Check sheet for the drawn part. Datum: minimum x, y, z corner. Units: mm. A direction names the side the tool comes from. Give positions to 0.01 mm unless a question says otherwise; leave off trailing zeros. Loops run counter-clockwise (first coordinate to the right, second up) from the corner with the lowest first, then second, coordinate; pieces in that order, holes last. Notation, with made-up numbers: (86, 39.5) - (121, 39.5) arc R19 cw to (121, 66.5) - close; hole circle Ø4 at (-26.5, -9). An arc over 180 degrees is marked (long way). Use a Markdown table: item, result. Add a question column.
1. Cross-section at C-C on y = 3.5. Enter the section's corners in (x, z).
2. Depth check by flat-ended pin: P1, Ø2, axis at y = 17, z = 12.5, coming from the -X side; P2, Ø1, axis at y = 8.5, z = 3, coming from the -X side; P3, Ø2, axis at y = 11.5, z = 20, coming from the +X side. Enter the tip coordinate at first touch or a pass-through.
3. Material ranges on L1, parallel to Z at x = 13.97, y = 9.75; L2, parallel to Y at x = 1.5, z = 10.75; L3, parallel to Z at x = 7.5, y = 19.5, recorded low to high.
4. Cross-section at B-B on x = 13.97. Enter the section's corners in (y, z).
5. Cross-section at A-A on z = 13.97. Enter the section's corners in (x, y), and give its area (3 significant figures).
6. Set-up check for the marked faces 4 and 5: record each of +Z, -Z, +X, -X, +Y, -Y from which the full face is reachable in a straight line by a thin tool's end or side.
7. Draft check along X on the marked faces 1, 2 and 3. Enter one of: pulls with the +X half, pulls with the -X half, needs draft (parallel to the pull), parting line crosses it, or undercut.
8. Cross-section at D-D on x = 25. Enter the section's corners in (y, z).
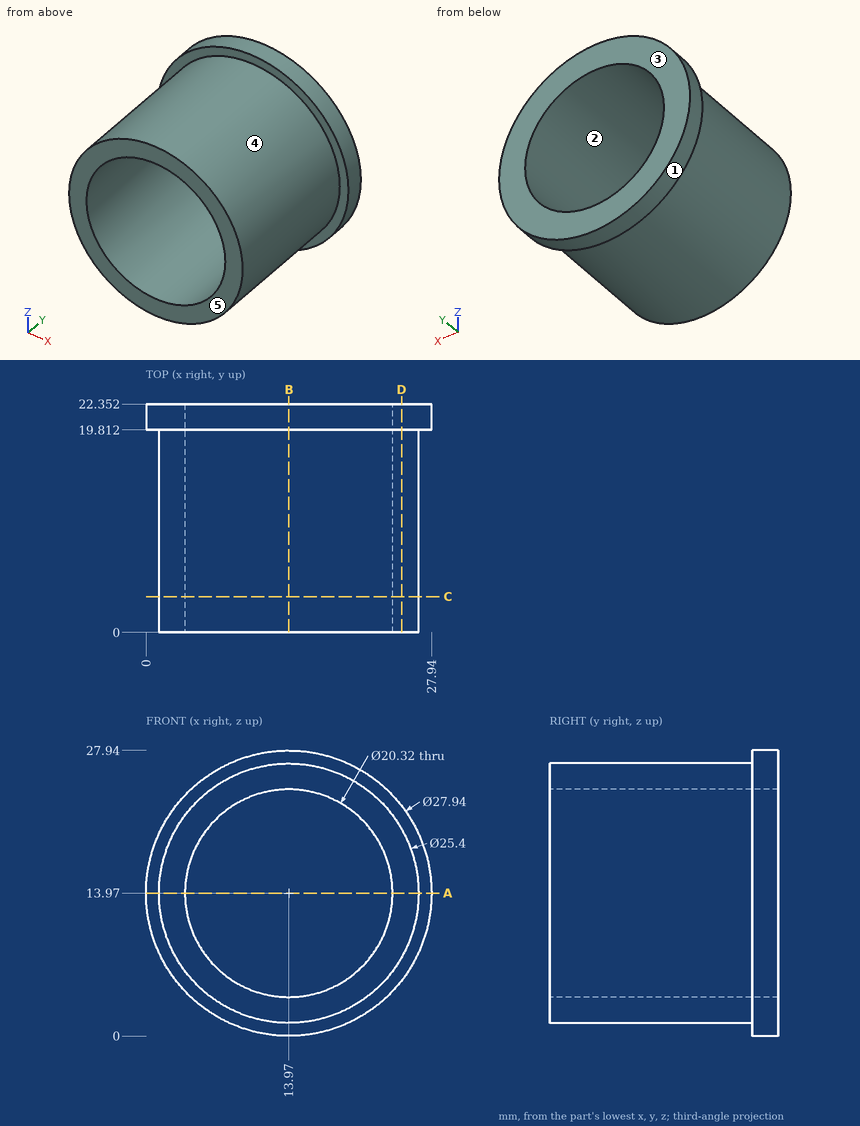
Values found:
| question | item | result |
|---|---|---|
| 1 | outline | circle Ø25.4 at (13.97, 13.97); hole circle Ø20.32 at (13.97, 13.97) |
| 2 | P1 | stops at x = 1.28 |
| 2 | P2 | stops at x = 6.78 |
| 2 | P3 | stops at x = 25.63 |
| 3 | L1 | z = 1.27 to 3.81, 24.13 to 26.67 |
| 3 | L2 | y = 19.81 to 22.35 |
| 3 | L3 | z = 3.04 to 6.14, 21.8 to 24.9 |
| 4 | outline | (0, 1.27) - (19.81, 1.27) - (19.81, 0) - (22.35, 0) - (22.35, 3.81) - (0, 3.81) - close; (0, 24.13) - (22.35, 24.13) - (22.35, 27.94) - (19.81, 27.94) - (19.81, 26.67) - (0, 26.67) - close |
| 5 | outline | (0, 19.81) - (1.27, 19.81) - (1.27, 0) - (3.81, 0) - (3.81, 22.35) - (0, 22.35) - close; (24.13, 0) - (26.67, 0) - (26.67, 19.81) - (27.94, 19.81) - (27.94, 22.35) - (24.13, 22.35) - close |
| 5 | area | 120 mm2 |
| 6 | face 4 | -Y |
| 6 | face 5 | +Z, -Z, +X, -X, -Y |
| 7 | face 1 | parting line crosses it |
| 7 | face 2 | undercut |
| 7 | face 3 | needs draft |
| 8 | outline | (0, 7.67) - (19.81, 7.67) - (19.81, 5.4) - (22.35, 5.4) - (22.35, 22.54) - (19.81, 22.54) - (19.81, 20.27) - (0, 20.27) - close |
